Could you check a few things on this model? Use its own coordinates, in mm. Face numbers are marked on the shaded views. A direction names the side the tool comes from. Coordinates: 2 decimals unless noted, no trailing zeros. Order: outer loops, then holes, each group sorted by start corner. A loop starts at its lowest first (then second) coordinate and runs counter-clockwise, first axis right, second up. Notation, with made-up numbers: (86, 74.25) -> (99, 74.25) arc R6 cw to (99, 84.25) -> close; hole circle Ø4 at (-12, 25.5). An arc over 180 degrees is marked (long way). Put each result on its own line as item: value. Start each with the question number.
Q1. If we section it at C-C (z = 3): Please give me the cut outline in (x, y) (3 decimals), and give its area (3 significant figures).
Q2. Please list where these lines run through material, in increasing order: line 1 along Y through (x, z) = (0, 3.8) (3 decimals); line 2 along Z through (x, y) = (3.25, 5.5); line 3 along Z through (x, y) = (-3.75, 2).
Q3. Will these pins go through, and if not, where does the flat tip stop? pin 1 (5 mm diameter, centred on x = 0, y = 0, fed in from -Z); pin 2 (1.5 mm diameter, centred on x = 8, z = 2, fed in from +Y); pin 3 (6 mm diameter, centred on x = 8.5, y = 6.5, fed in from +Z); pin 4 (2 mm diameter, centred on x = 2, z = 2.5, fed in from +Y).
Q4. We'd pull the mould along X, two halves only. Please class the marked faces 1, 2 and 3: +X half, -X half, draft (parallel to the pull), parting line (faces both ways), or undercut.
Q5. For the marked faces 4 and 5, which set-ups out of +Z, -Z, +X, -X, +Y, -Y let a thin tool reach every point of the face, with its end or its side?
Q6. If we section it at A-A (y = 0): Please give me the cut outline in (x, z) (3 decimals), and give its area (3 significant figures).
from build123d import *

# Parameters (mm, degrees)
F0_R     = 11
F1_DEPTH = 2
F2_R     = 6
F3_DEPTH = 0.5
F4_R     = 4.075
F5_DEPTH = 3.75
F6_R     = 3
F7_DEPTH = 5.08
F8_R     = 0.5


with BuildPart() as f1:
    # F0 (on Top) → F1 (new body)
    with BuildSketch(Plane.XY):
        Circle(F0_R)
    extrude(amount=F1_DEPTH)

    # F2 (on face) → F3 (join)
    with BuildSketch(Plane.XY.offset(2)):
        Circle(F2_R)
    extrude(amount=F3_DEPTH)

    # F4 (on face) → F5 (join)
    with BuildSketch(Plane.XY.offset(2.5)):
        Circle(F4_R)
    extrude(amount=F5_DEPTH)

    # F6 (on face) → F7 (cut)
    with BuildSketch(Plane.XY.offset(6.25)):
        Circle(F6_R)
    extrude(amount=-F7_DEPTH, mode=Mode.SUBTRACT)

    # F8
    f8_edges = [f1.edges().sort_by_distance(p)[0] for p in [
        (-11, 0, 2),
        (-11, 0, 0),
    ]]
    fillet(f8_edges, radius=F8_R)


solid = f1.part
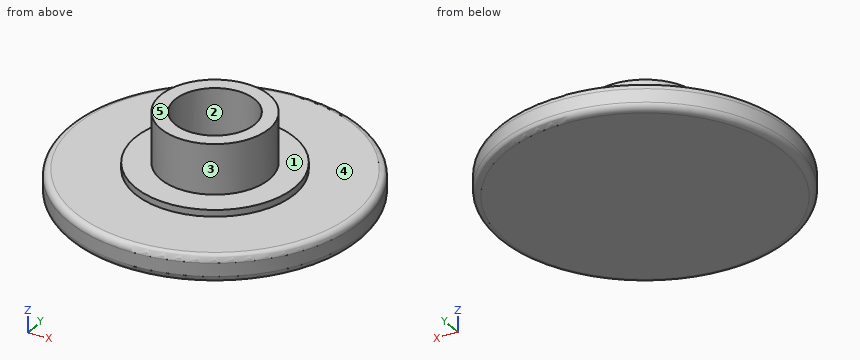
The answers:
1. outline: circle Ø8.15 at (0, 0); hole circle Ø6 at (0, 0)
1. area: 23.9 mm^2
2. line 1: -4.075 to -3, 3 to 4.075
2. line 2: 0 to 2
2. line 3: 0 to 2.5
3. pin 1: z = 0
3. pin 2: y = 8.17
3. pin 3: z = 2
3. pin 4: y = 10.88
4. face 1: draft
4. face 2: undercut
4. face 3: parting line
5. face 4: +Z
5. face 5: +Z, +X, -X, +Y, -Y
6. outline: (-11, 0.5) arc R0.5 ccw to (-10.5, 0) -> (10.5, 0) arc R0.5 ccw to (11, 0.5) -> (11, 1.5) arc R0.5 ccw to (10.5, 2) -> (6, 2) -> (6, 2.5) -> (4.075, 2.5) -> (4.075, 6.25) -> (3, 6.25) -> (3, 1.17) -> (-3, 1.17) -> (-3, 6.25) -> (-4.075, 6.25) -> (-4.075, 2.5) -> (-6, 2.5) -> (-6, 2) -> (-10.5, 2) arc R0.5 ccw to (-11, 1.5) -> close
6. area: 49.9 mm^2
